Source: CAD feature listing. Evaluate the final solid. Frame: model axes, mm. Face numbers are marked on the shaded views. Give positions to 0.01 mm unless a question says otherwise; leave off trailing zeros. Write each loop counter-clockwise with the first axis right and the second up, starting at its lowest first coordinate (ties: lowest second). Pieces come first, ordered by that corner, then holes.
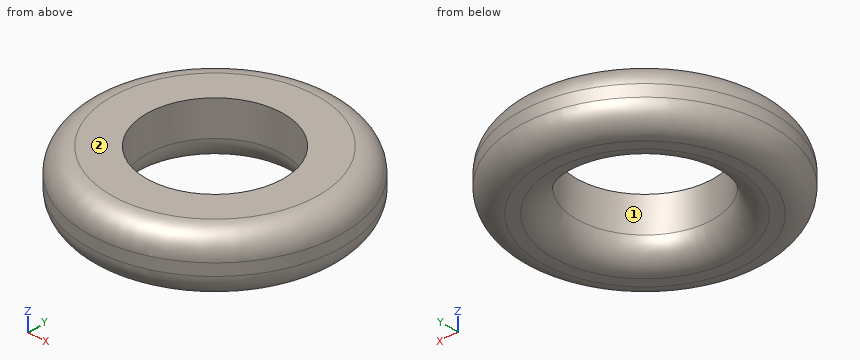
```python
from build123d import *

# Parameters (mm, degrees)
SKETCH1_R           = 3.25
SKETCH1_R_2         = 1.75
BOSS_EXTRUDE1_DEPTH = 1.5
FILLET1_R           = 0.6


with BuildPart() as part:
    # Sketch1 → Boss-Extrude1 (new body)
    with BuildSketch(Plane.XY):
        Circle(SKETCH1_R)
        Circle(SKETCH1_R_2, mode=Mode.SUBTRACT)
    extrude(amount=BOSS_EXTRUDE1_DEPTH)

    # Fillet1
    fillet1_edges = [part.edges().sort_by_distance(p)[0] for p in [
        (-3.25, 0, 0),
        (-3.25, 0, 1.5),
        (-1.75, 0, 0),
    ]]
    fillet(fillet1_edges, radius=FILLET1_R)


solid = part.part
```
1. Section query A-A (y = 0). Return loops of the section in (x, z), plus the area to 3 significant figures.
2. Pull-direction query (Y, two-part tool) for the marked faces 1 and 2; classes: pulls with the +Y half, pulls with the -Y half, needs draft (parallel to the pull), parting line crosses it, or undercut.
3. Pin query (flat end, axial travel): P1, Ø2, axis at x = 2, y = 2.5, coming from the +Z side. Return the tip coordinate at first contact, or that it passes through.
4. Section query D-D (z = 1.35). Return loops of the section in (x, y), plus the area to 3 significant figures.
5. Line query: probe 1 along Z at (x, y) = (-1.5, 2.25); probe 2 along Y at (x, z) = (0, 0.9); probe 3 along Y at (x, z) = (0.5, 1.4). Output: solid intervals per line, ascending.
6. Section query C-C (z = 0.2). Return loops of the section in (x, y).
The answers:
1. outline: (-3.25, 0.6) arc R0.6 ccw to (-2.65, 0) - (-2.35, 0) arc R0.6 ccw to (-1.75, 0.6) - (-1.75, 1.5) - (-2.65, 1.5) arc R0.6 ccw to (-3.25, 0.9) - close; (1.75, 0.6) arc R0.6 ccw to (2.35, 0) - (2.65, 0) arc R0.6 ccw to (3.25, 0.6) - (3.25, 0.9) arc R0.6 ccw to (2.65, 1.5) - (1.75, 1.5) - close
1. area: 4.04 mm2
2. face 1: undercut
2. face 2: needs draft
3. P1: stops at z = 1.5
4. outline: circle Ø6.09 at (0, 0); hole circle Ø3.5 at (0, 0)
4. area: 19.5 mm2
5. probe 1: z = 0 to 1.5
5. probe 2: y = -3.25 to -1.75, 1.75 to 3.25
5. probe 3: y = -2.94 to -1.68, 1.68 to 2.94
6. outline: circle Ø6.19 at (0, 0); hole circle Ø3.81 at (0, 0)
